from build123d import *

# Parameters (mm, degrees)
SKETCH1_W            = 190
SKETCH1_H            = 50
BASE_DEPTH           = 0.8
SKETCH2_W            = 10
SKETCH2_H            = 10
SWITCHES_DEPTH       = 10
M5_CLEARANCE_HOLE1_D = 5.5


with BuildPart() as part:
    # Sketch1 → Base (new body, symmetric)
    with BuildSketch(Plane(origin=(0, 0, 0), x_dir=(1, 0, 0), z_dir=(0, 1, 0))):
        Rectangle(SKETCH1_W, SKETCH1_H)
    extrude(amount=BASE_DEPTH, both=True)

    # Sketch2 → Switches (add)
    with BuildSketch(Plane(origin=(0, 0.8, 0), x_dir=(1, 0, 0), z_dir=(0, 1, 0))):
        with Locations((-62, 0)):
            Rectangle(SKETCH2_W, SKETCH2_H)
        with Locations((-75, 13)):
            Rectangle(SKETCH2_W, SKETCH2_H)
        with Locations((-75, -13)):
            Rectangle(SKETCH2_W, SKETCH2_H)
        with Locations((-88, 0)):
            Rectangle(SKETCH2_W, SKETCH2_H)
        with Locations((-25, 10)):
            Rectangle(SKETCH2_W, SKETCH2_H)
        with Locations((25, 10)):
            Rectangle(SKETCH2_W, SKETCH2_H)
        with Locations((88, 0)):
            Rectangle(SKETCH2_W, SKETCH2_H)
        with Locations((75, -13)):
            Rectangle(SKETCH2_W, SKETCH2_H)
        with Locations((62, 0)):
            Rectangle(SKETCH2_W, SKETCH2_H)
        with Locations((75, 13)):
            Rectangle(SKETCH2_W, SKETCH2_H)
    extrude(amount=SWITCHES_DEPTH)

    # M5 Clearance Hole1 (through all)
    with Locations(Plane(origin=(0, 0.8, 0), x_dir=(1, 0, 0), z_dir=(0, 1, 0))):
        with Locations((-44, 0), (44, 0)):
            Hole(M5_CLEARANCE_HOLE1_D / 2)


solid = part.part
Part model, mm, in its own coordinate system. A direction names the side the tool comes from. Round coordinates to 2 decimals unless told otherwise and drop trailing zeros. Loops run counter-clockwise (first coordinate to the right, second up) from the corner with the lowest first, then second, coordinate; pieces in that order, holes last. Notation, with made-up numbers: (77, -2.75) - (131, -2.75) arc R20 ccw to (131, 9.25) - close; hole circle Ø4 at (-14.5, 89). An arc over 180 degrees is marked (long way). Answer as a JSON object with one key per item and string values.
Item 1: Pull direction X, two halves, no side cores. Call faces 4 (the face through (62, 6, -5)), 5 (the face through (-80, 6, -13)), 6 (the face through (20, 6, -10)): pulls with the +X half, pulls with the -X half, needs draft (parallel to the pull), parting line crosses it, or undercut.
Output:
{"face 4": "needs draft", "face 5": "pulls with the -X half", "face 6": "undercut"}
Item 2: Band-saw the part on C-C on y = 7. State how many separate pieces and enclosed holes the cut face has, plus the area to 3 significant figures.
Output:
{"separate pieces": "10", "enclosed holes": "0", "area": "1,000 mm2"}
Item 3: Band-saw the part on A-A on x = 44. List the corners of the cut face in (y, z).
Output:
{"outline": "(-0.8, -25) - (0.8, -25) - (0.8, -2.75) - (-0.8, -2.75) - close; (-0.8, 2.75) - (0.8, 2.75) - (0.8, 25) - (-0.8, 25) - close"}
Item 4: Band-saw the part on B-B on z = 0. List the corners of the cut face in (x, y).
Output:
{"outline": "(-95, -0.8) - (-46.75, -0.8) - (-46.75, 0.8) - (-57, 0.8) - (-57, 10.8) - (-67, 10.8) - (-67, 0.8) - (-83, 0.8) - (-83, 10.8) - (-93, 10.8) - (-93, 0.8) - (-95, 0.8) - close; (-41.25, -0.8) - (41.25, -0.8) - (41.25, 0.8) - (-41.25, 0.8) - close; (46.75, -0.8) - (95, -0.8) - (95, 0.8) - (93, 0.8) - (93, 10.8) - (83, 10.8) - (83, 0.8) - (67, 0.8) - (67, 10.8) - (57, 10.8) - (57, 0.8) - (46.75, 0.8) - close"}
Item 5: Pin check, flat tips, straight feed: pin 1 (3 mm diameter, centred on y = 4, z = -15.5, fed in from -X); pin 2 (3 mm diameter, centred on y = 7.5, z = 2.5, fed in from +X); pin 3 (3 mm diameter, centred on x = 75, y = 4.5, fed in from +Z); pin 4 (5 mm diameter, centred on x = -44, z = 0, fed in from -Y). Stop position of each tip, or through.
Output:
{"pin 1": "x = -80", "pin 2": "x = 93", "pin 3": "z = 18", "pin 4": "through"}
Item 6: Wall check: L1, parallel to X at y = 6, z = 3.5; L2, parallel to X at y = 3.75, z = -6.5; L3, parallel to Z at x = -44, y = -0.3. Give the ranges that are in metal, low to high.
Output:
{"L1": "-93 to -83, -67 to -57, 57 to 67, 83 to 93", "L2": "-30 to -20, 20 to 30", "L3": "-25 to -2.75, 2.75 to 25"}
Item 7: Band-saw the part on D-D on x = -38. List the corners of the cut face in (y, z), plus the area to 3 significant figures.
Output:
{"outline": "(-0.8, -25) - (0.8, -25) - (0.8, 25) - (-0.8, 25) - close", "area": "80.0 mm2"}
Item 8: Tool access for faces 1 (the face through (25, 6, -5)), 2 (the face through (-75, 6, -8)), 3 (the face through (-80, 6, 13)): list every direction of +Z, -Z, +X, -X, +Y, -Y with a clear straight run to the whole face (end or side of a thin tool).
Output:
{"face 1": "+Z, +Y", "face 2": "-X, +Y", "face 3": "+Z, -Z, -X, +Y"}
